```python
from build123d import *

# Parameters (mm, degrees)
SKETCH1_W                      = 300
SKETCH1_H                      = 85
BASE_FLANGE2_DEPTH             = 3
EDGE_FLANGE1_STRIP_W           = 13.4732
EDGE_FLANGE1_STRIP_H           = 3
EDGE_FLANGE1_STRIP_CUT_DEPTH   = 300
EDGE_FLANGE1_STRIP_2_W         = 13.4732
EDGE_FLANGE1_STRIP_2_H         = 3
EDGE_FLANGE1_STRIP_CUT_2_DEPTH = 300
EDGE_FLANGE1_DEPTH             = 300
EDGE_FLANGE1_BEND_DEPTH        = 300
SKETCH17_R                     = 3
CUT_EXTRUDE1_DEPTH             = 10


# Sheet-metal steps are written as plain solids
with BuildPart() as part:
    # Sketch1 → Base-Flange2 (new body)
    with BuildSketch(Plane(origin=(0, 0, 0), x_dir=(1, 0, 0), z_dir=(0, 1, 0))):
        Rectangle(SKETCH1_W, SKETCH1_H)
    extrude(amount=-BASE_FLANGE2_DEPTH)

    # Edge-Flange1 strip (across the edge) → Edge-Flange1 strip cut (cut)
    with BuildSketch(Plane(origin=(-150, 0, 42.5), x_dir=(0, 0, -1), z_dir=(1, 0, 0))):
        with Locations((-3, -1.5)):
            Rectangle(EDGE_FLANGE1_STRIP_W, EDGE_FLANGE1_STRIP_H)
    extrude(amount=EDGE_FLANGE1_STRIP_CUT_DEPTH, mode=Mode.SUBTRACT)

    # Edge-Flange1 strip 2 (across the edge) → Edge-Flange1 strip cut 2 (cut)
    with BuildSketch(Plane(origin=(150, 0, -42.5), x_dir=(0, 0, 1), z_dir=(-1, 0, 0))):
        with Locations((-3, -1.5)):
            Rectangle(EDGE_FLANGE1_STRIP_2_W, EDGE_FLANGE1_STRIP_2_H)
    extrude(amount=EDGE_FLANGE1_STRIP_CUT_2_DEPTH, mode=Mode.SUBTRACT)

    # Edge-Flange1 section (across the edge) → Edge-Flange1 (add)
    with BuildSketch(Plane(origin=(-150, 0, 42.5), x_dir=(0, 0, -1), z_dir=(1, 0, 0))):
        with BuildLine():
            Line((0, 0.7366), (0, 117))
            Line((0, 117), (3, 117))
            Line((3, 117), (3, 0.7366))
            ThreePointArc((3, 0.7366), (3.215745145, 0.215745145), (3.7366, 0))
            Line((3.7366, 0), (3.7366, -3))
            ThreePointArc((3.7366, -3), (1.094424801, -1.905575199), (0, 0.7366))
        make_face()
    extrude(amount=EDGE_FLANGE1_DEPTH)

    # Edge-Flange1 section 2 (across the edge) → Edge-Flange1 bend (add)
    with BuildSketch(Plane(origin=(150, 0, -42.5), x_dir=(0, 0, 1), z_dir=(-1, 0, 0))):
        with BuildLine():
            Line((0, 0.7366), (0, 117))
            Line((0, 117), (3, 117))
            Line((3, 117), (3, 0.7366))
            ThreePointArc((3, 0.7366), (3.215745145, 0.215745145), (3.7366, 0))
            Line((3.7366, 0), (3.7366, -3))
            ThreePointArc((3.7366, -3), (1.094424801, -1.905575199), (0, 0.7366))
        make_face()
    extrude(amount=EDGE_FLANGE1_BEND_DEPTH)

    # Sketch17 → Cut-Extrude1 (cut)
    with BuildSketch(Plane(origin=(0, 0, 0), x_dir=(1, 0, 0), z_dir=(0, 1, 0))):
        with Locations(Location((-125, 24.5, 0), (0, 0, 270))):
            Circle(SKETCH17_R)
        with Locations(Location((-125, -20.5, 0), (0, 0, 270))):
            Circle(SKETCH17_R)
        with Locations(Location((125, 24.5, 0), (0, 0, 270))):
            Circle(SKETCH17_R)
        with Locations(Location((125, -20.5, 0), (0, 0, 270))):
            Circle(SKETCH17_R)
    extrude(amount=-CUT_EXTRUDE1_DEPTH, mode=Mode.SUBTRACT)


solid = part.part
```
Part model, mm, in its own coordinate system. A direction names the side the tool comes from. Round coordinates to 2 decimals unless told otherwise and drop trailing zeros. Loops run counter-clockwise (first coordinate to the right, second up) from the corner with the lowest first, then second, coordinate; pieces in that order, holes last.
Item 1: Cut at C-C, the plane y = 7.5. Give the cut face in (x, z).
Item 2: Mould opens along X. For faces 1 (the face through (-2, -3, -1)), 2 (the face through (127.974, -1.479, -24.891)), 3 (the face through (-150, -0.5, 0.2)) say: +X half, -X half, draft (parallel to the pull), parting line (faces both ways), or undercut.
Item 3: Cut at D-D, the plane x = -43. Give the cut face in (y, z), then the cut area to 3 significant figures.
Item 4: Cut at A-A, the plane x = -125. Give the cut face in (y, z), then the cut area to 3 significant figures.
Item 5: Drop a flat-ended pin along its axis: P1, Ø23.5, axis at x = -70, z = -10, coming from the +Y side. Give the stop position or say it passes through.
Item 6: Cut at B-B, the plane z = -24.5. Give the cut face in (x, y).
Item 7: 3-axis set-ups, long thin cutter, end or side, ignore diameter. For faces 4 (the face through (-2, 0, -1)), 5 (the face through (150, -0.5, 0.2)): which of +Z, -Z, +X, -X, +Y, -Y reach the whole face in a straight line?
Item 8: Drill centre lines: line 1 (X direction, y = -2, z = 20); line 2 (Z direction, x = 63.5, y = 8.5); line 3 (Y direction, x = 105, z = -29.5). Where is each one in solid material? Low to high.
A:
1. outline: (-150, -42.5) - (150, -42.5) - (150, -39.5) - (-150, -39.5) - close; (-150, 39.5) - (150, 39.5) - (150, 42.5) - (-150, 42.5) - close
2. face 1: draft
2. face 2: undercut
2. face 3: -X half
3. outline: (-3, -38.76) arc R3.74 ccw to (0.74, -42.5) - (117, -42.5) - (117, -39.5) - (0.74, -39.5) arc R0.74 cw to (0, -38.76) - (0, 38.76) arc R0.74 cw to (0.74, 39.5) - (117, 39.5) - (117, 42.5) - (0.74, 42.5) arc R3.74 ccw to (-3, 38.76) - close
3. area: 951 mm2
4. outline: (-3, -38.76) arc R3.74 ccw to (0.74, -42.5) - (117, -42.5) - (117, -39.5) - (0.74, -39.5) arc R0.74 cw to (0, -38.76) - (0, -27.5) - (-3, -27.5) - close; (-3, -21.5) - (0, -21.5) - (0, 17.5) - (-3, 17.5) - close; (-3, 23.5) - (0, 23.5) - (0, 38.76) arc R0.74 cw to (0.74, 39.5) - (117, 39.5) - (117, 42.5) - (0.74, 42.5) arc R3.74 ccw to (-3, 38.76) - close
4. area: 915 mm2
5. P1: stops at y = 0
6. outline: (-150, -3) - (-128, -3) - (-128, 0) - (-150, 0) - close; (-122, -3) - (122, -3) - (122, 0) - (-122, 0) - close; (128, -3) - (150, -3) - (150, 0) - (128, 0) - close
7. face 4: +X, -X, +Y
7. face 5: +Z, -Z, +X, +Y, -Y
8. line 1: x = -150 to -127.96, -122.04 to 122.04, 127.96 to 150
8. line 2: z = -42.5 to -39.5, 39.5 to 42.5
8. line 3: y = -3 to 0
